Could you check a few things on this model? Use its own coordinates, in mm. A direction names the side the tool comes from. Coordinates: 2 decimals unless noted, no trailing zeros. Loops run counter-clockwise (first coordinate to the right, second up) from the corner with the lowest first, then second, coordinate; pieces in that order, holes last. Notation, with made-up numbers: M 44.25,11.5 L 52.25,11.5 A27 ccw 52.25,42.5 Z; hole C 63,65 d11. An arc over 180 degrees is marked long. Return JSON: item names as keys, results as strings. Group by question number.
from build123d import *

# Parameters (mm, degrees)
F1_DEPTH = 15
F2_R     = 2.125
F3_DEPTH = 25
F4_SIZE  = 5
F5_R     = 7.5
F6_R     = 2.25
F7_DEPTH = 25
F9_DEPTH = 4


# Not quite as in the source:
# - a feature names something its author has since deleted; it is built from what else it names


with BuildPart() as f1:
    # F0 (on Top) → F1 (new body)
    with BuildSketch(Plane.XY):
        Polygon((-16.7, 0), (0, 0), (16.7, 0), (16.7, 14.2), (37.5, 14.2), (37.5, 19.2), (13.5, 19.2), (13.5, 3.2), (0, 3.2), (-13.5, 3.2), (-26.1, 3.2), (-26.1, -15), (-20.1, -15), (-20.1, 0), align=None)
    extrude(amount=F1_DEPTH)

    # F2 (on face) → F3 (cut)
    with BuildSketch(Plane.XZ):
        with Locations((0, 7.5)):
            Circle(F2_R)
        with Locations((30, 7.5)):
            Circle(F2_R)
    extrude(amount=-F3_DEPTH, mode=Mode.SUBTRACT)

    # F4
    f4_edges = [f1.edges().sort_by_distance(p)[0] for p in [
        (16.7, 14.2, 7.5),
    ]]
    chamfer(f4_edges, length=F4_SIZE)

    # F5
    f5_edges = [f1.edges().sort_by_distance(p)[0] for p in [
        (37.5, 16.7, 15),
        (-23.1, -15, 15),
    ]]
    fillet(f5_edges, radius=F5_R)

    # F6 (on face) → F7 (cut)
    with BuildSketch(Plane.YZ.offset(-20.1)):
        with Locations((-7.5, 8.5048094716)):
            Circle(F6_R)
    extrude(amount=-F7_DEPTH, mode=Mode.SUBTRACT)

    # F8 (on face) → F9 (cut)
    with BuildSketch(Plane.YZ.offset(-20.1)):
        Polygon((-3.0775, 5.9514779061), (-3.0775, 11.0581410371), (-7.5, 13.6114726026), (-11.9225, 11.0581410371), (-11.9225, 5.9514779061), (-7.5, 3.3981463406), align=None)
    extrude(amount=-F9_DEPTH, mode=Mode.SUBTRACT)


solid = f1.part
(1) We'd pull the mould along Y, two halves only. Please class faces 6 (the face through (-22.072, -9.68, 12.353)), 7 (the face through (19.2, 11.7, 7.4)), 8 (the face through (16.7, 5, 7)): +Y half, -Y half, draft (parallel to the pull), parting line (faces both ways), or undercut.
(2) Imagine slicing it at D-D, the plane x = 6.5. Write out the boundary of the cut face in (y, z), then the cut area to 3 significant figures.
(3) Imagine slicing it at A-A, the plane x = 0. Write out the boundary of the cut face in (y, z) (3 decimals), then the cut area to 3 significant figures.
(4) Imagine slicing it at B-B, the plane z = 2.5. Write out the boundary of the cut face in (x, y), then the cut area to 3 significant figures.
(5) For faces 1 (the face through (27.7, 14.2, 7.4)), 2 (the face through (13.5, 11, 7)), 3 (the face through (-24.1, -10, 7)), 4 (the face through (37.5, 17, 4)), 5 (the face through (-23, -15, 4)), which set-ups out of +Z, -Z, +X, -X, +Y, -Y let a thin tool reach every point of the face, with its end or its side?
(6) Imagine slicing it at C-C, the plane y = -6.5. Write out the boundary of the cut face in (x, z).
(7) If I drill on L1, parallel to Z at x = 30, y = 16 (3 decimals); L2, parallel to Y at x = 22.5, z = 5.75; L3, parallel to Y at x = -3, z = 12, over which ranges is the centre line in solid material (lowest first)? Write a range as [from, to].
(8) Will these pins go through, and if not, where does the flat tip stop? P1, Ø8, axis at y = 7.5, z = 8, coming from the -X side; P2, Ø6, axis at x = 3.5, z = 12, coming from the +Y side; P3, Ø4.5, axis at x = -8, z = 7.5, coming from the -Y side.
Checks:
{
 "1": {"face 6": "undercut", "face 7": "-Y half", "face 8": "draft"},
 "2": {"outline": "M 0,0 L 3.2,0 L 3.2,15 L 0,15 Z", "area": "48.0 mm²"},
 "3": {"outline": "M 0,0 L 3.2,0 L 3.2,5.375 L 0,5.375 Z; M 0,9.625 L 3.2,9.625 L 3.2,15 L 0,15 Z", "area": "34.4 mm²"},
 "4": {"outline": "M -26.1,-15 L -20.1,-15 L -20.1,0 L 16.7,0 L 16.7,9.2 L 21.7,14.2 L 37.5,14.2 L 37.5,19.2 L 13.5,19.2 L 13.5,3.2 L -26.1,3.2 Z", "area": "395 mm²"},
 "5": {"face 1": "+Z, -Z, +X, -Y", "face 2": "+Z, -Z, -X, +Y", "face 3": "+X", "face 4": "+Z, -Z, +X, +Y, -Y", "face 5": "+Z, -Z, +X, -X, -Y"},
 "6": {"outline": "M -26.1,0 L -20.1,0 L -20.1,3.98 L -24.1,3.98 L -24.1,6.49 L -26.1,6.49 Z; M -26.1,10.52 L -24.1,10.52 L -24.1,13.03 L -20.1,13.03 L -20.1,15 L -26.1,15 Z"},
 "7": {"L1": "[0, 5.375], [9.625, 15]", "L2": "[14.2, 19.2]", "L3": "[0, 3.2]"},
 "8": {"P1": "x = 13.5", "P2": "y = 3.2", "P3": "y = 0"}
}
